Can you work these out from the drawing? Everything is in mm from the part's minimum corner. A direction names the side the tool comes from. Round coordinates to 2 decimals unless told otherwise and drop trailing zeros. Loops run counter-clockwise (first coordinate to the right, second up) from the corner with the lowest first, then second, coordinate; pieces in that order, holes last. Notation, with made-up numbers: M -30.75,12 L 1.25,12 A10 cw 1.25,16 Z; hole C 89,64 d5. An arc over 180 degrees is marked long. Answer in a Markdown table with one row per item.
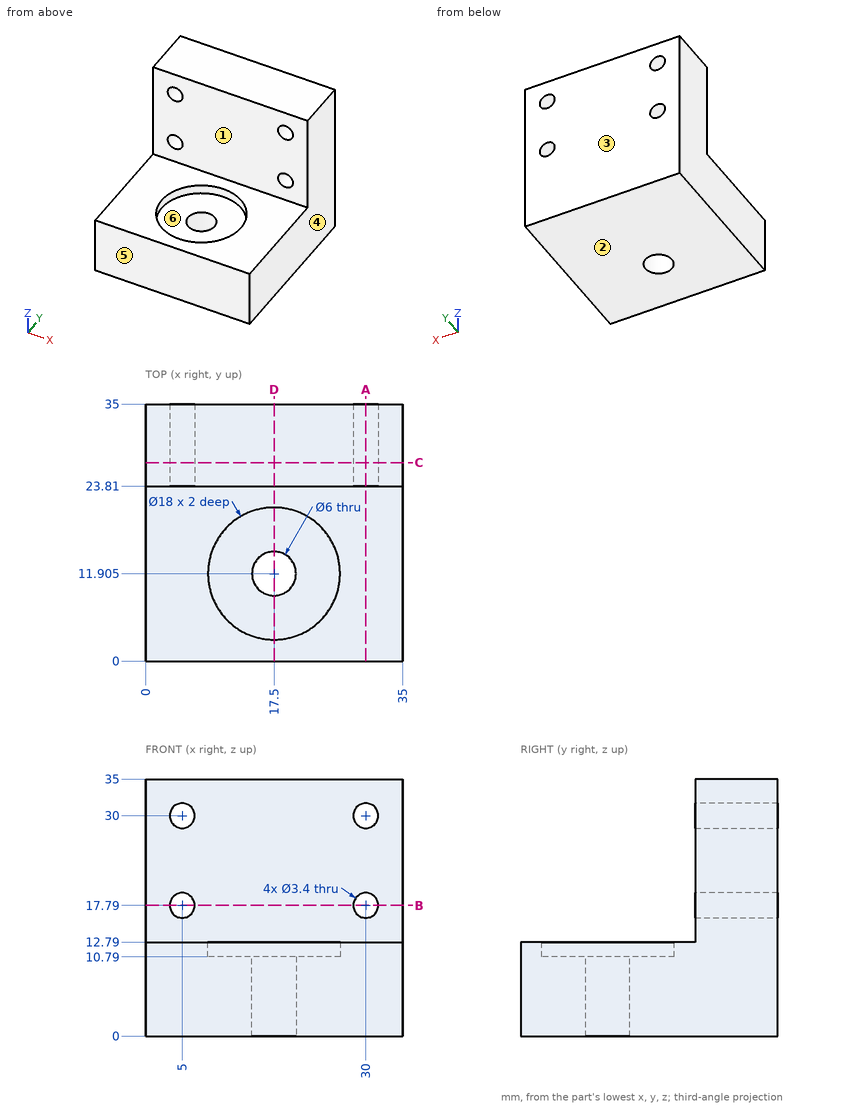
1) If we mould it in two halves opening along Y, with no side actions, what happens to the marked faces 3, 4, 5 and 6? For each: released by +Y, released by -Y, zero draft, split by the parting line, or undercut.
Computed:
| item | result |
|---|---|
| face 3 | released by +Y |
| face 4 | zero draft |
| face 5 | released by -Y |
| face 6 | undercut |
2) I want a section at C-C, the plane y = 27. Please give me the cut outline in (x, z), plus the area to 3 significant figures.
Computed:
| item | result |
|---|---|
| outline | M 0,0 L 35,0 L 35,35 L 0,35 Z; hole C 5,17.79 d3.4; hole C 5,30 d3.4; hole C 30,17.79 d3.4; hole C 30,30 d3.4 |
| area | 1,190 mm² |
3) I want a section at B-B, the plane z = 17.79. Please give me the cut outline in (x, y).
Computed:
| item | result |
|---|---|
| outline | M 0,23.81 L 3.3,23.81 L 3.3,35 L 0,35 Z; M 6.7,23.81 L 28.3,23.81 L 28.3,35 L 6.7,35 Z; M 31.7,23.81 L 35,23.81 L 35,35 L 31.7,35 Z |
4) I want a section at A-A, the plane x = 30. Please give me the cut outline in (y, z).
Computed:
| item | result |
|---|---|
| outline | M 0,0 L 35,0 L 35,16.09 L 23.81,16.09 L 23.81,12.79 L 0,12.79 Z; M 23.81,19.49 L 35,19.49 L 35,28.3 L 23.81,28.3 Z; M 23.81,31.7 L 35,31.7 L 35,35 L 23.81,35 Z |
5) I need wall thicknesses on line 1 (X direction, y = 28.5, z = 30); line 2 (Y direction, x = 17.5, z = 12) (3 decimals); line 3 (X direction, y = 33, z = 31.5). Which ranges of each line are inside material? Lowest first, please.
Computed:
| item | result |
|---|---|
| line 1 | x = 0 to 3.3, 6.7 to 28.3, 31.7 to 35 |
| line 2 | y = 0 to 2.905, 20.905 to 35 |
| line 3 | x = 0 to 4.2, 5.8 to 29.2, 30.8 to 35 |
6) Will these pins go through, and if not, where does the flat tip stop? P1, Ø1, axis at x = 11.5, y = 7, coming from the +Z side; P2, Ø19, axis at x = 21, y = 9, coming from the +Z side; P3, Ø11, axis at x = 13.5, z = 19, coming from the -Y side.
Computed:
| item | result |
|---|---|
| P1 | stops at z = 10.79 |
| P2 | stops at z = 12.79 |
| P3 | stops at y = 23.81 |
7) Which directions (+Z, -Z, +X, -X, +Y, -Y) give clear straight access to the entire face, cutting with the end or side of a thin tool? Please do the marked faces 1 and 2.
Computed:
| item | result |
|---|---|
| face 1 | +Z, +X, -X, -Y |
| face 2 | -Z, +X, -X, +Y, -Y |
8) I want a section at D-D, the plane x = 17.5. Please give me the cut outline in (y, z) (3 decimals).
Computed:
| item | result |
|---|---|
| outline | M 0,0 L 8.905,0 L 8.905,10.79 L 2.905,10.79 L 2.905,12.79 L 0,12.79 Z; M 14.905,0 L 35,0 L 35,35 L 23.81,35 L 23.81,12.79 L 20.905,12.79 L 20.905,10.79 L 14.905,10.79 Z |
